```python
from build123d import *

# Parameters (mm, degrees)
BOSS_EXTRUDE1_DEPTH  = 2.7
FILLET1_R            = 5
BOSS_EXTRUDE2_DEPTH  = 2
FILLET2_R            = 5
FILLET3_R            = 1
FASTENER_HOLES_DEPTH = 52.527686738
FILLET4_R            = 1
WEDGE_DEPTH          = 2.7
CUT_EXTRUDE2_DEPTH   = 53.103914951


with BuildPart() as part:
    # Sketch1 → Boss-Extrude1 (new body)
    with BuildSketch(Plane.XY):
        Polygon((-20.75, -5.5), (20.75, -5.5), (20.75, -24.5), (45.25, -24.5), (45.25, -5.5), (45.25, 5.5), (-45.25, 5.5), (-45.25, -5.5), (-45.25, -24.5), (-20.75, -24.5), align=None)
    extrude(amount=-BOSS_EXTRUDE1_DEPTH)

    # Fillet1
    fillet1_edges = [part.edges().sort_by_distance(p)[0] for p in [
        (-45.25, 5.5, -1.35),
        (45.25, 5.5, -1.35),
    ]]
    fillet(fillet1_edges, radius=FILLET1_R)

    # Sketch2 → Boss-Extrude2 (add)
    with BuildSketch(Plane.XY):
        with BuildLine():
            Line((-25, 5.5), (25, 5.5))
            Line((25, 5.5), (25, 2.5))
            ThreePointArc((25, 2.5), (0, 4.06865167), (-25, 2.5))
            Line((-25, 2.5), (-25, 5.5))
        make_face()
    extrude(amount=BOSS_EXTRUDE2_DEPTH)

    # Fillet2
    # the kernel refuses this fillet: 5 mm, written as the material it takes off along each edge
    with BuildSketch(Plane(origin=(-25, 2.5, 0), x_dir=(0, 1, 0), z_dir=(0, 0, 1))) as fillet2_piece_1:
        with BuildLine():
            CenterArc((5.522601094, -4.316999388), FILLET2_R, 120.299508601, 65.491069006)
            ThreePointArc((0.548114523, -4.821462818), (0.288680447, -2.409069013), (0, 0))
            Line((0, 0), (3, 0))
        make_face()
    extrude(amount=14.131295591, mode=Mode.SUBTRACT)
    with BuildSketch(Plane(origin=(25, 2.5, 0), x_dir=(-0.9936001438850942, 0.11295465493515582, 0), z_dir=(0, 0, 1))) as fillet2_piece_2:
        with BuildLine():
            CenterArc((4.913174714, -4.999632066), FILLET2_R, 90.695089087, 65.491069006)
            Line((0.338863965, -2.980800432), (0, 0))
            ThreePointArc((0, 0), (2.426259118, -0.014717375), (4.852518236, 0))
        make_face()
    extrude(amount=14.131295591, mode=Mode.SUBTRACT)

    # Fillet3
    # the kernel refuses this fillet: 1 mm, written as the material it adds along each edge
    with BuildSketch(Plane(origin=(20.683000612, 8.022601094, 0), x_dir=(-0.10089268591027718, -0.9948973142640452, 0), z_dir=(-0.9948973142640452, 0.10089268591027718, 0))) as fillet3_piece_1_section:
        with BuildLine():
            CenterArc((5 + FILLET3_R, FILLET3_R), FILLET3_R, 180, 90)
            Line((5, FILLET3_R), (5, 0))
            Line((5, 0), (5 + FILLET3_R, 0))
        make_face()
    fillet3_piece_1 = revolve(axis=Axis((20.683000612, 8.022601094, 0), (0, 0, 1)), revolution_arc=94.145051676, mode=Mode.PRIVATE)
    fillet3_piece_1 = split(fillet3_piece_1, bisect_by=Plane(origin=(23.299245225, 5.5, 0.284698162), z_dir=(0, -1, 0)), keep=Keep.TOP, mode=Mode.PRIVATE)
    add(fillet3_piece_1)
    with BuildSketch(Plane(origin=(0, -195.93134833, 0), x_dir=(0.1008926859104223, 0.9948973142640303, 0), z_dir=(0.9948973142640303, -0.1008926859104223, 0))) as fillet3_piece_2:
        with BuildLine():
            CenterArc((200 - FILLET3_R, FILLET3_R), FILLET3_R, 270, 90)
            Line((200, FILLET3_R), (200, 0))
            Line((200, 0), (200 - FILLET3_R, 0))
        make_face()
    revolve(axis=Axis((0, -195.93134833, 0), (0, 0, 1)), revolution_arc=11.581155214)
    with BuildSketch(Plane(origin=(-20.683000612, 8.022601094, 0), x_dir=(-0.999587613586136, -0.028715897429362498, 0), z_dir=(-0.028715897429362498, 0.999587613586136, 0))) as fillet3_piece_3_section:
        with BuildLine():
            CenterArc((5 + FILLET3_R, FILLET3_R), FILLET3_R, 180, 90)
            Line((5, FILLET3_R), (5, 0))
            Line((5, 0), (5 + FILLET3_R, 0))
        make_face()
    fillet3_piece_3 = revolve(axis=Axis((-20.683000612, 8.022601094, 0), (0, 0, 1)), revolution_arc=94.145051676, mode=Mode.PRIVATE)
    fillet3_piece_3 = split(fillet3_piece_3, bisect_by=Plane(origin=(-23.299245227, 5.5, 0.284698166), z_dir=(0, -1, 0)), keep=Keep.TOP, mode=Mode.PRIVATE)
    add(fillet3_piece_3)
    # the kernel refuses this fillet: 1 mm, written as the material it takes off along each edge
    with BuildSketch(Plane(origin=(20.683000612, 8.022601094, 2), x_dir=(0.9995876135861396, -0.028715897429238708, 0), z_dir=(0.028715897429238708, 0.9995876135861396, 0))) as fillet3_2_piece_1:
        with BuildLine():
            CenterArc((5 - FILLET3_R, FILLET3_R), FILLET3_R, 270, 90)
            Line((5, FILLET3_R), (5, 0))
            Line((5, 0), (5 - FILLET3_R, 0))
        make_face()
    revolve(axis=Axis((20.683000612, 8.022601094, 2), (0, 0, -1)), revolution_arc=94.145051676, mode=Mode.SUBTRACT)
    with BuildSketch(Plane(origin=(0, -195.93134833, 2), x_dir=(0.10089268591041367, 0.9948973142640313, 0), z_dir=(0.9948973142640313, -0.10089268591041367, 0))) as fillet3_2_piece_2:
        with BuildLine():
            CenterArc((200 + FILLET3_R, -FILLET3_R), FILLET3_R, 90, 90)
            Line((200, -FILLET3_R), (200, 0))
            Line((200, 0), (200 + FILLET3_R, 0))
        make_face()
    revolve(axis=Axis((0, -195.93134833, 2), (0, 0, 1)), revolution_arc=11.581155214, mode=Mode.SUBTRACT)
    with BuildSketch(Plane(origin=(-20.683000612, 8.022601094, 2), x_dir=(0.10089268591039939, -0.9948973142640327, 0), z_dir=(0.9948973142640327, 0.10089268591039939, 0))) as fillet3_2_piece_3:
        with BuildLine():
            CenterArc((5 - FILLET3_R, FILLET3_R), FILLET3_R, 270, 90)
            Line((5 - FILLET3_R, 0), (5, 0))
            Line((5, 0), (5, FILLET3_R))
        make_face()
    revolve(axis=Axis((-20.683000612, 8.022601094, 2), (0, 0, -1)), revolution_arc=94.145051676, mode=Mode.SUBTRACT)
    with BuildSketch(Plane(origin=(-27.5, 5.5, 2), x_dir=(0, 0, -1), z_dir=(1, 0, 0))) as fillet3_2_piece_4:
        with BuildLine():
            CenterArc((FILLET3_R, -FILLET3_R), FILLET3_R, 90, 90)
            Line((0, -FILLET3_R), (0, 0))
            Line((0, 0), (FILLET3_R, 0))
        make_face()
    extrude(amount=55, mode=Mode.SUBTRACT)

    # Sketch3 → Fastener holes (cut, through all)
    with BuildSketch(Plane.XY):
        with BuildLine():
            Line((-33.25, -24.5), (-33.25, -21.5))
            ThreePointArc((-33.25, -21.5), (-30.25, -18.5), (-27.25, -21.5))
            Line((-27.25, -21.5), (-27.25, -24.5))
            ThreePointArc((-27.25, -24.5), (-30.25, -27.5), (-33.25, -24.5))
        make_face()
        with BuildLine():
            Line((30.65, -24.5), (30.65, -21.5))
            ThreePointArc((30.65, -21.5), (27.65, -18.5), (24.65, -21.5))
            Line((24.65, -21.5), (24.65, -24.5))
            ThreePointArc((24.65, -24.5), (27.65, -27.5), (30.65, -24.5))
        make_face()
    extrude(amount=-FASTENER_HOLES_DEPTH, mode=Mode.SUBTRACT)

    # Fillet4
    fillet4_edges = [part.edges().sort_by_distance(p)[0] for p in [
        (-27.25, -24.5, -1.35),
        (-33.25, -24.5, -1.35),
        (30.65, -24.5, -1.35),
        (24.65, -24.5, -1.35),
    ]]
    fillet(fillet4_edges, radius=FILLET4_R)

    # Sketch4 → Wedge (add)
    with BuildSketch(Plane.XY):
        Polygon((45.25, -12), (45.905097241, -24.5), (45.25, -24.5), align=None)
        Polygon((-45.25, -12), (-45.25, -24.5), (-45.905097241, -24.5), align=None)
    extrude(amount=-WEDGE_DEPTH)

    # Sketch5 → Cut-Extrude2 (cut, through all)
    with BuildSketch(Plane.XY):
        Polygon((43.905097241, -24.5), (43.25, -12), (41.905097241, -12), (41.905097241, -24.5), align=None)
        Polygon((-41.905097241, -24.5), (-43.905097241, -24.5), (-43.25, -12), (-41.905097241, -12), align=None)
    extrude(amount=-CUT_EXTRUDE2_DEPTH, mode=Mode.SUBTRACT)


solid = part.part
```
Read the model definition and answer for the solid it produces. Units are mm, in the model's axes. A direction names the side the tool comes from. Coordinates: 2 decimals unless noted, no trailing zeros. Loops run counter-clockwise (first coordinate to the right, second up) from the corner with the lowest first, then second, coordinate; pieces in that order, holes last. Notation, with made-up numbers: (-13.5, -38.5) - (18.5, -38.5) arc R27 ccw to (18.5, -2.5) - close; hole circle Ø9 at (10, 43). An arc over 180 degrees is marked (long way). Answer in a Markdown table with one row per item.
1. Find section A-A, the plane y = -8.5. Write down the section's boundary in (x, z), then the cut area to 3 significant figures.
Conclusion:
| item | result |
|---|---|
| outline | (-45.25, -2.7) - (-20.75, -2.7) - (-20.75, 0) - (-45.25, 0) - close; (20.75, -2.7) - (45.25, -2.7) - (45.25, 0) - (20.75, 0) - close |
| area | 132 mm² |
2. Which of the six approach directions +Z, -Z, +X, -X, +Y, -Y give full straight-line access (tool end or side, diameter ignored) to faces 5 (the face through (24.65, -22, -1)), 6 (the face through (43.82, 4, -1.37))?
Conclusion:
| item | result |
|---|---|
| face 5 | +Z, -Z, -Y |
| face 6 | +Z, -Z, +X, +Y |
3. Determine the mould class of faces 1 (the face through (-43.582, -18.338, -1.331)), 2 (the face through (0, -5.5, -1)), 3 (the face through (45, -24.5, -1)), 4 (the face through (45.25, -6, -1)) for opening direction X: +X half, -X half, draft (parallel to the pull), parting line (faces both ways), or undercut.
Conclusion:
| item | result |
|---|---|
| face 1 | undercut |
| face 2 | undercut |
| face 3 | draft |
| face 4 | +X half |
4. Straight lines are drawn through the part: line 1 (X direction, y = -14, z = -1.75); line 2 (X direction, y = -13.5, z = -1.9); line 3 (Y direction, x = -40.5, z = -1.9). For each, find the intervals that lie inside material, in ascending order.
Conclusion:
| item | result |
|---|---|
| line 1 | x = -45.35 to -43.35, -41.91 to -20.75, 20.75 to 41.91, 43.35 to 45.35 |
| line 2 | x = -45.33 to -43.33, -41.91 to -20.75, 20.75 to 41.91, 43.33 to 45.33 |
| line 3 | y = -24.5 to 5.49 |
5. Given pin 1 (9 mm diameter, centred on x = 16.5, y = -13.5, fed in from +Z); pin 2 (1 mm diameter, centred on y = -22.5, z = -2, fed in from -X); pin 3 (1.1 mm diameter, centred on x = -42.5, z = -2, fed in from -Y), each flat-ended and moving along its own axis, determine where each tip first touches the part or whether it passes through.
Conclusion:
| item | result |
|---|---|
| pin 1 | stops at z = 0 |
| pin 2 | stops at x = -45.83 |
| pin 3 | stops at y = -12 |
6. Find section D-D, the plane x = -30.25. Write down the section's boundary in (y, z), then the cut area to 3 significant figures.
Conclusion:
| item | result |
|---|---|
| outline | (-18.5, -2.7) - (5.5, -2.7) - (5.5, 0) - (-18.5, 0) - close |
| area | 64.8 mm² |
7. Find section B-B, the plane y = -16. Write down the section's boundary in (x, z).
Conclusion:
| item | result |
|---|---|
| outline | (-45.46, -2.7) - (-43.46, -2.7) - (-43.46, 0) - (-45.46, 0) - close; (-41.91, -2.7) - (-20.75, -2.7) - (-20.75, 0) - (-41.91, 0) - close; (20.75, -2.7) - (41.91, -2.7) - (41.91, 0) - (20.75, 0) - close; (43.46, -2.7) - (45.46, -2.7) - (45.46, 0) - (43.46, 0) - close |
